Geometry: final body of the model. Coordinates: model frame, mm. Give positions to 0.01 mm unless a question says otherwise; leave off trailing zeros. One line per item, written item: value. Start each with the question number.
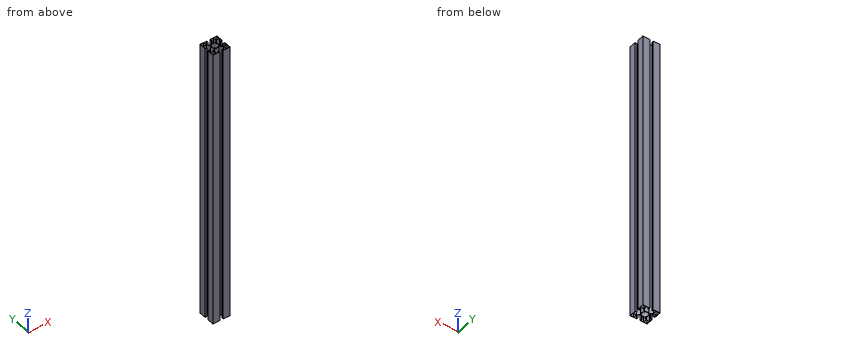
from build123d import *

# Parameters (mm, degrees)
ESBO_O1_W                = 9
ESBO_O1_H                = 9
ESBO_O1_R                = 8
RESSALTO_EXTRUS_O4_DEPTH = 734.5


with BuildPart() as part:
    # Esboço1 → Ressalto-extrusão4 (new body)
    with BuildSketch(Plane.XY):
        with BuildLine():
            Line((-4.5, 22.5), (-22.5, 22.5))
            Line((-22.5, 22.5), (-22.5, 4.5))
            Line((-22.5, 4.5), (-17.5, 4.5))
            Line((-17.5, 4.5), (-17.5, 5))
            Line((-17.5, 5), (-22, 5))
            Line((-22, 5), (-22, 12.5))
            Line((-22, 12.5), (-13.207106781, 12.5))
            Line((-13.207106781, 12.5), (-6.707685904, 6.000579123))
            ThreePointArc((-6.707685904, 6.000579123), (-9, 0), (-6.707685904, -6.000579123))
            Line((-6.707685904, -6.000579123), (-13.207106781, -12.5))
            Line((-13.207106781, -12.5), (-22, -12.5))
            Line((-22, -12.5), (-22, -5))
            Line((-22, -5), (-17.5, -5))
            Line((-17.5, -5), (-17.5, -4.5))
            Line((-17.5, -4.5), (-22.5, -4.5))
            Line((-22.5, -4.5), (-22.5, -22.5))
            Line((-22.5, -22.5), (-4.5, -22.5))
            Line((-4.5, -22.5), (-4.5, -17.5))
            Line((-4.5, -17.5), (-5, -17.5))
            Line((-5, -17.5), (-5, -22))
            Line((-5, -22), (-12.5, -22))
            Line((-12.5, -22), (-12.5, -13.207106781))
            Line((-12.5, -13.207106781), (-6.000579123, -6.707685904))
            ThreePointArc((-6.000579123, -6.707685904), (0, -9), (6.000579123, -6.707685904))
            Line((6.000579123, -6.707685904), (12.5, -13.207106781))
            Line((12.5, -13.207106781), (12.5, -22))
            Line((12.5, -22), (5, -22))
            Line((5, -22), (5, -17.5))
            Line((5, -17.5), (4.5, -17.5))
            Line((4.5, -17.5), (4.5, -22.5))
            Line((4.5, -22.5), (22.5, -22.5))
            Line((22.5, -22.5), (22.5, -4.5))
            Line((22.5, -4.5), (17.5, -4.5))
            Line((17.5, -4.5), (17.5, -5))
            Line((17.5, -5), (22, -5))
            Line((22, -5), (22, -12.5))
            Line((22, -12.5), (13.207106781, -12.5))
            Line((13.207106781, -12.5), (6.707685904, -6.000579123))
            ThreePointArc((6.707685904, -6.000579123), (9, 0), (6.707685904, 6.000579123))
            Line((6.707685904, 6.000579123), (13.207106781, 12.5))
            Line((13.207106781, 12.5), (22, 12.5))
            Line((22, 12.5), (22, 5))
            Line((22, 5), (17.5, 5))
            Line((17.5, 5), (17.5, 4.5))
            Line((17.5, 4.5), (22.5, 4.5))
            Line((22.5, 4.5), (22.5, 22.5))
            Line((22.5, 22.5), (4.5, 22.5))
            Line((4.5, 22.5), (4.5, 17.5))
            Line((4.5, 17.5), (5, 17.5))
            Line((5, 17.5), (5, 22))
            Line((5, 22), (12.5, 22))
            Line((12.5, 22), (12.5, 13.207106781))
            Line((12.5, 13.207106781), (6.000579123, 6.707685904))
            ThreePointArc((6.000579123, 6.707685904), (0, 9), (-6.000579123, 6.707685904))
            Line((-6.000579123, 6.707685904), (-12.5, 13.207106781))
            Line((-12.5, 13.207106781), (-12.5, 22))
            Line((-12.5, 22), (-5, 22))
            Line((-5, 22), (-5, 17.5))
            Line((-5, 17.5), (-4.5, 17.5))
            Line((-4.5, 17.5), (-4.5, 22.5))
        make_face()
        with Locations((17.5, 17.5)):
            Rectangle(ESBO_O1_W, ESBO_O1_H, mode=Mode.SUBTRACT)
        with Locations((-17.5, -17.5)):
            Rectangle(ESBO_O1_W, ESBO_O1_H, mode=Mode.SUBTRACT)
        with Locations((17.5, -17.5)):
            Rectangle(ESBO_O1_W, ESBO_O1_H, mode=Mode.SUBTRACT)
        with Locations((-17.5, 17.5)):
            Rectangle(ESBO_O1_W, ESBO_O1_H, mode=Mode.SUBTRACT)
        Circle(ESBO_O1_R, mode=Mode.SUBTRACT)
    extrude(amount=RESSALTO_EXTRUS_O4_DEPTH)


solid = part.part
Item 1: Pin query (flat end, axial travel): pin 1 (1.5 mm diameter, centred on x = -2.5, z = 385.5, fed in from -Y); pin 2 (1 mm diameter, centred on x = -9.5, y = 7, fed in from -Z). Return the tip coordinate at first contact, or that it passes through.
Item 2: Ray query, line 1 along X through (y, z) = (20, 687); line 2 along X through (y, z) = (14, 310). Return the intervals inside material, ascending. Write a range as [from, to].
Item 3: Section A-A, the plane z = 573. State how many separate pieces and enclosed holes the cut face has, then the cut area to 3 significant figures.
Geometry check:
1. pin 1: stops at y = -8.83
1. pin 2: passes through
2. line 1: x = [-22.5, -22], [-13, -12.5], [-5, -4.5], [4.5, 5], [12.5, 13], [22, 22.5]
2. line 2: x = [-22.5, -22], [-13, -12.5], [12.5, 13], [22, 22.5]
3. separate pieces: 1
3. enclosed holes: 5
3. area: 215 mm2
